Autodesk Inventor part; units mm, degrees
ref_plane "YZ Plane" through (0, 0, 0) normal (1, 0, 0) x (0, 1, 0)
ref_plane "XZ Plane" through (0, 0, 0) normal (0, 1, 0) x (-1, 0, 0)
ref_plane "XY Plane" through (0, 0, 0) normal (0, 0, 1) x (1, 0, 0)
sketch "Sketch1" plane through (0, 0, 0) normal (0, 1, 0) x (-1, 0, 0)
  line L0 (170, 275) -> (0, 275)
  line L1 (0, 275) -> (0, -275)
  line L2 (0, -275) -> (170, -275)
  line L3 (170, -275) -> (170, 275)
  line L4 (170, 255) -> (0, 255)
  line L5 (170, -255) -> (0, -255)
  point P0 (0, 0)
  point P1 (0, 0)
  dimension "d0" = 170
  dimension "d1" = 550
  dimension "d4" = 20
  dimension "d5" = 20
extrude "Extrusion1" add sketch "Sketch1" along normal blind 3
extrude "Extrusion2" add sketch "Sketch1" along normal blind 3.1 contours L3 L4 L1 L0 | L3 L2 L1 L5
equation "\"d1\" = track_width"
equation "\"d4\" = curb_width"
equation "\"d5\" = curb_width"
equation "\"d2\" = track_height"
equation "\"d6\" = track_height + curb_height"
properties part number "intersection_extension"
Here's how the part is built. I have some questions about the finished solid (model axes, mm). Coordinates: 2 decimals unless noted, no trailing zeros. Write each loop counter-clockwise with the first axis right and the second up, starting at its lowest first coordinate (ties: lowest second). Pieces come first, ordered by that corner, then holes.
Item 1: If I drill on line 1 (Y direction, x = -143, z = -62), over which ranges is the centre line in solid material (lowest first)?
Item 2: I want a section at B-B on z = 27.5. Write out the boundary of the cut face in (x, y), and give its area (3 significant figures).
Item 3: I want a section at A-A on x = -70.5. Write out the boundary of the cut face in (y, z).
Item 4: Will this pin go through, and if not, where does the flat tip stop? pin 1 (8 mm diameter, centred on x = -82.5, z = 18, fed in from +Y).
Findings below:
1. line 1: y = 0 to 3
2. outline: (-170, 0) - (0, 0) - (0, 3) - (-170, 3) - close
2. area: 510 mm2
3. outline: (0, -275) - (3.1, -275) - (3.1, -255) - (3, -255) - (3, 255) - (3.1, 255) - (3.1, 275) - (0, 275) - close
4. pin 1: stops at y = 3
